```python
from build123d import *

# Parameters (mm, degrees)
SKETCH1_R           = 12.7
BOSS_EXTRUDE1_DEPTH = 457.2
SKETCH2_R           = 3.175
BOSS_EXTRUDE2_DEPTH = 25.4
CUT_EXTRUDE1_START  = -50.8
SKETCH3_R           = 3.175
CUT_EXTRUDE1_DEPTH  = 50.8


with BuildPart() as part:
    # Sketch1 → Boss-Extrude1 (new body)
    with BuildSketch(Plane(origin=(0, 0, 0), x_dir=(0, 0, -1), z_dir=(1, 0, 0))):
        Circle(SKETCH1_R)
    extrude(amount=BOSS_EXTRUDE1_DEPTH)

    # Sketch2 → Boss-Extrude2 (add)
    with BuildSketch(Plane.ZY):
        with BuildLine():
            Line((-38.1, -101.6), (38.1, -101.6))
            ThreePointArc((38.1, -101.6), (56.060512242, -94.160512242), (63.5, -76.2))
            Line((63.5, -76.2), (63.5, 76.2))
            ThreePointArc((63.5, 76.2), (56.060512242, 94.160512242), (38.1, 101.6))
            Line((38.1, 101.6), (-38.1, 101.6))
            ThreePointArc((-38.1, 101.6), (-56.060512242, 94.160512242), (-63.5, 76.2))
            Line((-63.5, 76.2), (-63.5, -76.2))
            ThreePointArc((-63.5, -76.2), (-56.060512242, -94.160512242), (-38.1, -101.6))
        make_face()
        Circle(SKETCH2_R, mode=Mode.SUBTRACT)
        with BuildLine():
            Line((31.75, 76.2), (-31.75, 76.2))
            ThreePointArc((-31.75, 76.2), (-36.240128061, 74.340128061), (-38.1, 69.85))
            Line((-38.1, 69.85), (-38.1, 38.1))
            Line((-38.1, 38.1), (38.1, 38.1))
            Line((38.1, 38.1), (38.1, 69.85))
            ThreePointArc((38.1, 69.85), (36.240128061, 74.340128061), (31.75, 76.2))
        make_face(mode=Mode.SUBTRACT)
        with BuildLine():
            Line((31.75, -76.2), (-31.75, -76.2))
            ThreePointArc((-31.75, -76.2), (-36.240128061, -74.340128061), (-38.1, -69.85))
            Line((-38.1, -69.85), (-38.1, -38.1))
            Line((-38.1, -38.1), (38.1, -38.1))
            Line((38.1, -38.1), (38.1, -69.85))
            ThreePointArc((38.1, -69.85), (36.240128061, -74.340128061), (31.75, -76.2))
        make_face(mode=Mode.SUBTRACT)
    extrude(amount=BOSS_EXTRUDE2_DEPTH)

    # Sketch3 → Cut-Extrude1 (cut)
    with BuildSketch(Plane.ZY.offset(25.4).offset(CUT_EXTRUDE1_START)):
        Circle(SKETCH3_R)
    extrude(amount=CUT_EXTRUDE1_DEPTH, mode=Mode.SUBTRACT)


solid = part.part
```
Could you check a few things on this model? Use its own coordinates, in mm. A direction names the side the tool comes from. Round coordinates to 2 decimals unless told otherwise and drop trailing zeros. Write each loop counter-clockwise with the first axis right and the second up, starting at its lowest first coordinate (ties: lowest second). Pieces come first, ordered by that corner, then holes. Notation, with made-up numbers: M 53,-34 L 80,-34 A3 cw 80,-29 Z; hole C 13.5,25 d2. An arc over 180 degrees is marked long. Answer in a Markdown table with one row per item. Add a question column.
Q1. Will these pins go through, and if not, where does the flat tip stop? pin 1 Ø1 at (x, y) = (390, -14.5) entering from -Z; pin 2 Ø2 at (y, z) = (-32.5, 23) entering from +X.
Q2. Imagine slicing it at A-A (z = 20). Please give me the cut outline in (x, y).
Q3. If I drill on line 1 (Y direction, x = -13, z = 0) (3 decimals); line 2 (X direction, y = -69, z = -41.5); line 3 (Y direction, x = 13, z = 0) (3 decimals), over which ranges is the centre line in solid material (lowest first)? Write a range as from..to.
Q4. If we mould it in two halves opening along Y, with no side actions, what happens to faces 4 (the flat face through (-13, -101.6, -1)), 5 (the flat face through (-13, -54, 38.1)), 6 (the flat face through (-13, -1, 63.5))? For each: +Y half, -Y half, draft (parallel to the pull), parting line (faces both ways), or undercut.
Q5. On a 3-axis mill with a long thin cutter (end or side, diameter ignored), from which of +Z, -Z, +X, -X, +Y, -Y can I reach the whole of each face in a straight line? I mean faces 1 (the cylindrical face through (225.4, -12.4, 2.75)), 2 (the flat face through (-13, -38.1, -1)), 3 (the flat face through (-25.4, 1, 13)). Say none if no direction works.
Q6. Imagine slicing it at B-B (y = -44.5). Please give me the cut outline in (x, z).
Q7. Imagine slicing it at C-C (x = 296). Please give me the cut outline in (y, z).
Values:
| question | item | result |
|---|---|---|
| 1 | pin 1 | through |
| 1 | pin 2 | x = 0 |
| 2 | outline | M -25.4,-101.6 L 0,-101.6 L 0,-76.2 L -25.4,-76.2 Z; M -25.4,-38.1 L 0,-38.1 L 0,38.1 L -25.4,38.1 Z; M -25.4,76.2 L 0,76.2 L 0,101.6 L -25.4,101.6 Z |
| 3 | line 1 | -101.6..-76.2, -38.1..-3.175, 3.175..38.1, 76.2..101.6 |
| 3 | line 2 | -25.4..0 |
| 3 | line 3 | -12.7..-3.175, 3.175..12.7 |
| 4 | face 4 | -Y half |
| 4 | face 5 | undercut |
| 4 | face 6 | draft |
| 5 | face 1 | +X |
| 5 | face 2 | +X, -X |
| 5 | face 3 | +Z, -Z, -X, +Y, -Y |
| 6 | outline | M -25.4,-63.5 L 0,-63.5 L 0,-38.1 L -25.4,-38.1 Z; M -25.4,38.1 L 0,38.1 L 0,63.5 L -25.4,63.5 Z |
| 7 | outline | C 0,0 d25.4 |
